For this review, take the finished solid that the model builds, in its own axes (mm). Face numbers are marked on the shaded views. A direction names the side the tool comes from. Give positions to 0.01 mm unless a question says otherwise; leave off trailing zeros. Loops run counter-clockwise (first coordinate to the right, second up) from the corner with the lowest first, then second, coordinate; pieces in that order, holes last. Notation, with made-up numbers: (-5.5, -14) - (28.5, -14) arc R27 ccw to (28.5, 16) - close; hole circle Ø10 at (67, 17). An arc over 180 degrees is marked (long way). Answer in a Markdown table with one row per item.
```python
from build123d import *

# Parameters (mm, degrees)
F0_W      = 140
F0_H      = 70
F1_DEPTH  = 60
F2_R      = 20
F3_DEPTH  = 144.4
F4_W      = 30
F4_H      = 60
F5_DEPTH  = 30
F7_DEPTH  = 25
F8_R      = 30
F9_DEPTH  = 80
F10_R     = 20
F11_DEPTH = 80
F12_W     = 39.848283
F12_H     = 31.382198
F13_DEPTH = 80
F14_W     = 48.629179
F14_H     = 31.993205
F15_DEPTH = 80
F16_W     = 30
F16_H     = 60
F17_DEPTH = 30
F19_DEPTH = 10


with BuildPart() as f1:
    # F0 (on Top) → F1 (new body)
    with BuildSketch(Plane.XY):
        with Locations((-6.793272, 9.692355)):
            Rectangle(F0_W, F0_H)
    extrude(amount=F1_DEPTH)

    # F2 (on face) → F3 (cut)
    with BuildSketch(Plane.YZ.offset(63.206728)):
        with Locations((9.692355, 0)):
            Circle(F2_R)
    extrude(amount=-F3_DEPTH, mode=Mode.SUBTRACT)

    # F4 (on face) → F5 (cut)
    with BuildSketch(Plane.XY.offset(60)):
        with Locations((48.206728, 4.692355)):
            Rectangle(F4_W, F4_H)
    extrude(amount=-F5_DEPTH, mode=Mode.SUBTRACT)

    # F6 (on face) → F7 (cut)
    with BuildSketch(Plane.XZ.offset(-34.692355)):
        with BuildLine():
            ThreePointArc((53.206728, 45), (44.671194, 48.535534), (48.206728, 40))
            ThreePointArc((48.206728, 40), (51.742262, 41.464466), (53.206728, 45))
        make_face()
    extrude(amount=-F7_DEPTH, mode=Mode.SUBTRACT)

    # F8 (on face) → F9 (join)
    with BuildSketch(Plane(origin=(0, 44.692355, 0), x_dir=(-1, 0, 0), z_dir=(0, 1, 0))):
        with Locations((6.793272, 60)):
            Circle(F8_R)
    extrude(amount=-F9_DEPTH)

    # F10 (on face) → F11 (cut)
    with BuildSketch(Plane.XZ.offset(35.307645)):
        with Locations((-6.793272, 60)):
            Circle(F10_R)
    extrude(amount=-F11_DEPTH, mode=Mode.SUBTRACT)

    # F12 (on face) → F13 (cut)
    with BuildSketch(Plane.XZ.offset(35.307645)):
        with Locations((13.130869, 75.691099)):
            Rectangle(F12_W, F12_H)
    extrude(amount=-F13_DEPTH, mode=Mode.SUBTRACT)

    # F14 (on face) → F15 (cut)
    with BuildSketch(Plane.XZ.offset(35.307645)):
        with Locations((-31.107861, 75.996602)):
            Rectangle(F14_W, F14_H)
    extrude(amount=-F15_DEPTH, mode=Mode.SUBTRACT)

    # F16 (on face) → F17 (cut)
    with BuildSketch(Plane.XY.offset(60)):
        with Locations((-61.793272, 4.692355)):
            Rectangle(F16_W, F16_H)
    extrude(amount=-F17_DEPTH, mode=Mode.SUBTRACT)

    # F18 (on face) → F19 (cut)
    with BuildSketch(Plane.XZ.offset(-34.692355)):
        with BuildLine():
            ThreePointArc((-61.793272, 50), (-65.328806, 41.464466), (-56.793272, 45))
            ThreePointArc((-56.793272, 45), (-58.257738, 48.535534), (-61.793272, 50))
        make_face()
    extrude(amount=-F19_DEPTH, mode=Mode.SUBTRACT)


solid = f1.part
```
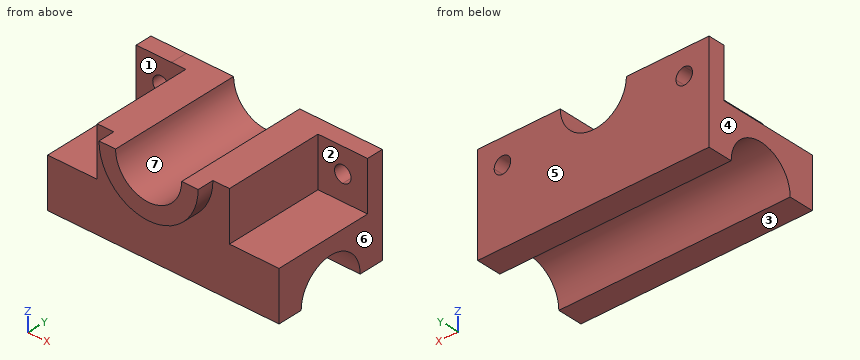
1. For the marked faces 1, 2 and 3, list the 3-axis set-ups (+Z, -Z, +X, -X, +Y, -Y) from which the entire face can be reached by the end or side of a thin tool; tool diameter is ignored.
Values:
| item | result |
|---|---|
| face 1 | +Z, -X, -Y |
| face 2 | +Z, +X, -Y |
| face 3 | -Z, +X, -X, +Y, -Y |
2. We need section D-D, the plane y = 6.5. Give the boundary of the cut face in (x, z).
Values:
| item | result |
|---|---|
| outline | (-76.79, 19.74) - (63.21, 19.74) - (63.21, 30) - (33.21, 30) - (33.21, 60) - (13.21, 60) arc R20 cw to (-26.79, 60) - (-46.79, 60) - (-46.79, 30) - (-76.79, 30) - close |
3. Wall thickness on line 1 (X direction, y = 42, z = 45); line 2 (Y direction, x = 28.5, z = 48); line 3 (X direction, y = 16.5, z = 34): over which ranges is each line inside the solid? List them lowest first. Write a range as [from, to].
Values:
| item | result |
|---|---|
| line 1 | x = [-76.79, -66.79], [-56.79, -20.02], [6.44, 43.21], [53.21, 63.21] |
| line 2 | y = [-25.31, 44.69] |
| line 3 | x = [-46.79, 33.21] |
4. We need section B-B, the plane z = 51.5. Give the boundary of the cut face in (x, y), and give its area (3 significant figures).
Values:
| item | result |
|---|---|
| outline | (-76.79, 34.69) - (-46.79, 34.69) - (-46.79, -25.31) - (-35.56, -25.31) - (-35.56, -35.31) - (-24.9, -35.31) - (-24.9, 44.69) - (-76.79, 44.69) - close; (11.31, -35.31) - (21.98, -35.31) - (21.98, -25.31) - (33.21, -25.31) - (33.21, 34.69) - (63.21, 34.69) - (63.21, 44.69) - (11.31, 44.69) - close |
| area | 3,880 mm^2 |
5. We need section A-A, the plane x = -52. Give the boundary of the cut face in (y, z).
Values:
| item | result |
|---|---|
| outline | (-25.31, 0) - (-10.31, 0) arc R20 cw to (29.69, 0) - (44.69, 0) - (44.69, 60) - (34.69, 60) - (34.69, 30) - (-25.31, 30) - close |
6. Clearance check with flat-ended pins moving along their axes: pin 1 (9 mm diameter, centred on x = 48.21, z = 45, fed in from -Y); pin 2 (2 mm diameter, centred on x = 3.5, y = -0.5, fed in from -Z) (3 decimals); pin 3 (12 mm diameter, centred on x = -45, z = 12.5, fed in from -Y); pin 4 (13 mm diameter, centred on x = -61.79, z = 45, fed in from +Y). State where each tip first meets the part, or that it passes through.
Values:
| item | result |
|---|---|
| pin 1 | passes through |
| pin 2 | stops at z = 16.575 |
| pin 3 | stops at y = -25.31 |
| pin 4 | stops at y = 44.69 |
7. We need section C-C, the plane y = -17.5. Give the boundary of the cut face in (x, z).
Values:
| item | result |
|---|---|
| outline | (-76.79, 0) - (63.21, 0) - (63.21, 30) - (33.21, 30) - (33.21, 60) - (13.21, 60) arc R20 cw to (-26.79, 60) - (-46.79, 60) - (-46.79, 30) - (-76.79, 30) - close |
8. Mouldability with a two-part tool opening along X and no side actions: class the marked faces 4, 5, 6 and 7 as released by +X, released by -X, zero draft, split by the parting line, or undercut.
Values:
| item | result |
|---|---|
| face 4 | released by -X |
| face 5 | zero draft |
| face 6 | released by +X |
| face 7 | undercut |
